Drawing for the job (mm, zero at the part's lowest x, y, z). A direction names the side the tool comes from. Give positions to 0.01 mm unless a question says otherwise; leave off trailing zeros. Loops run counter-clockwise (first coordinate to the right, second up) from the corner with the lowest first, then second, coordinate; pieces in that order, holes last. Notation, with made-up numbers: (28, 9.25) -> (78, 9.25) arc R24 ccw to (78, 32.25) -> close; hole circle Ø10 at (29.25, -34.5). An arc over 180 degrees is marked (long way). Use CSV: the item, a comma, the result in double quotes. Start each with the question number.
(1) Drill centre lines: probe 1 along X at (y, z) = (4.45, 6); probe 2 along X at (y, z) = (4.75, 25); probe 3 along X at (y, z) = (0.5, 15.5). Where is each one in solid material? Low to high.
(2) Flat gauge pins, fed straight in: pin 1 (3 mm diameter, centred on x = 10, z = 15.5, fed in from -Y); pin 2 (6 mm diameter, centred on x = 13.5, z = 18.5, fed in from +Y); pin 3 (1.5 mm diameter, centred on x = 13.5, y = 5, fed in from -Z); pin 4 (1 mm diameter, centred on x = 4, y = 5, fed in from +Z). Where does each tip first touch, or does it go through?
(3) Cut at C-C on z = 15.5. Write the cut outline in (x, y).
(4) Cut at B-B on y = 3.5. Write the cut outline in (x, z), then the cut area to 3 significant figures.
(5) 3-axis set-ups, long thin cutter, end or side, ignore diameter. For the marked faces 1 and 2: which of +Z, -Z, +X, -X, +Y, -Y reach the whole face in a straight line?
(6) Cut at D-D on x = 3. Write the cut outline in (y, z).
(7) Cut at A-A on x = 10. Write the cut outline in (y, z).
(8) Pull direction X, two halves, no side cores. Call the marked faces 3, 4, 5 and 6: pulls with the +X half, pulls with the -X half, needs draft (parallel to the pull), parting line crosses it, or undercut.
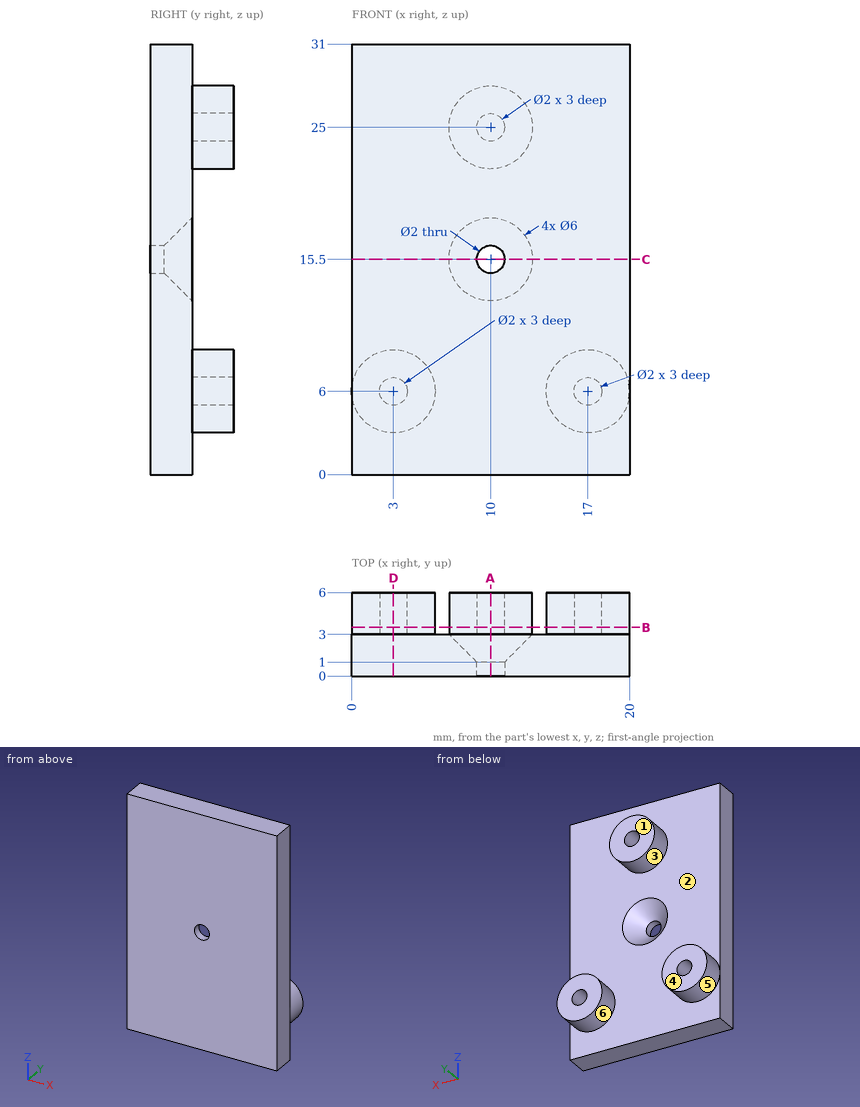
Check result:
1,probe 1,"0 to 2, 4 to 6, 14 to 16, 18 to 20"
1,probe 2,"7 to 9, 11 to 13"
1,probe 3,"0 to 9, 11 to 20"
2,pin 1,"y = 0"
2,pin 2,"y = 3"
2,pin 3,"z = 4.8"
2,pin 4,"z = 8.96"
3,outline,"(0, 0) -> (9, 0) -> (9, 1) -> (7, 3) -> (0, 3) -> close; (11, 0) -> (20, 0) -> (20, 3) -> (13, 3) -> (11, 1) -> close"
4,outline,"circle Ø6 at (3, 6); circle Ø6 at (10, 25); circle Ø6 at (17, 6); hole circle Ø2 at (3, 6); hole circle Ø2 at (10, 25); hole circle Ø2 at (17, 6)"
4,area,"75.4 mm²"
5,face 1,"+Z, -Z, +X, -X, +Y"
5,face 2,"+Y"
6,outline,"(0, 0) -> (3, 0) -> (3, 3) -> (6, 3) -> (6, 5) -> (3, 5) -> (3, 7) -> (6, 7) -> (6, 9) -> (3, 9) -> (3, 31) -> (0, 31) -> close"
7,outline,"(0, 0) -> (3, 0) -> (3, 12.5) -> (1, 14.5) -> (0, 14.5) -> close; (0, 16.5) -> (1, 16.5) -> (3, 18.5) -> (3, 22) -> (6, 22) -> (6, 24) -> (3, 24) -> (3, 26) -> (6, 26) -> (6, 28) -> (3, 28) -> (3, 31) -> (0, 31) -> close"
8,face 3,"parting line crosses it"
8,face 4,"needs draft"
8,face 5,"undercut"
8,face 6,"undercut"
